```python
from build123d import *

# Parameters (mm, degrees)
SKETCH1_R           = 30
SKETCH1_R_2         = 25
BOSS_EXTRUDE1_DEPTH = 109.9
SKETCH2_W           = 5
SKETCH2_H           = 6
CUT_EXTRUDE1_DEPTH  = 31
CHAMFER1_SIZE       = 0.5


with BuildPart() as part:
    # Sketch1 → Boss-Extrude1 (new body)
    with BuildSketch(Plane.XY):
        Circle(SKETCH1_R)
        Circle(SKETCH1_R_2, mode=Mode.SUBTRACT)
    extrude(amount=BOSS_EXTRUDE1_DEPTH)

    # Sketch2 → Cut-Extrude1 (cut, through all)
    with BuildSketch(Plane(origin=(0, 0, 0), x_dir=(0, 0, -1), z_dir=(1, 0, 0))):
        with Locations((-107.4, 0)):
            Rectangle(SKETCH2_W, SKETCH2_H)
    extrude(amount=CUT_EXTRUDE1_DEPTH, mode=Mode.SUBTRACT)

    # Chamfer1
    chamfer1_edges = [part.edges().sort_by_distance(p)[0] for p in [
        (-30, 0, 109.9),
        (-30, 0, 0),
    ]]
    chamfer(chamfer1_edges, length=CHAMFER1_SIZE)


solid = part.part
```
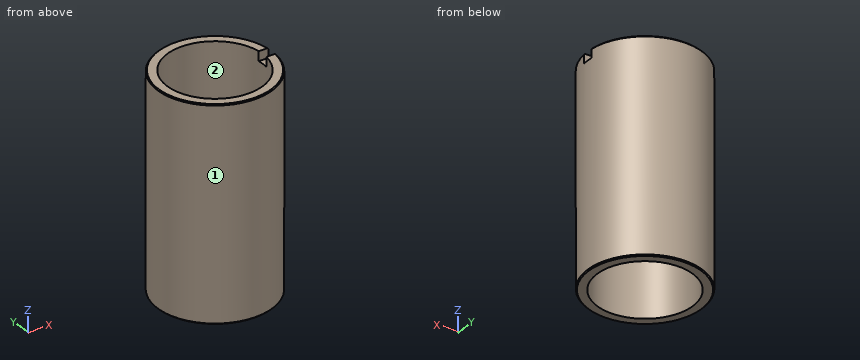
Source: CAD feature listing. Evaluate the final solid. Frame: model axes, mm. Face numbers are marked on the shaded views. Give positions to 0.01 mm unless a question says otherwise; leave off trailing zeros. Loops run counter-clockwise (first coordinate to the right, second up) from the corner with the lowest first, then second, coordinate; pieces in that order, holes last. Notation, with made-up numbers: (38.25, 24.25) -> (76.25, 24.25) arc R7 ccw to (76.25, 29.25) -> close; hole circle Ø8 at (81, 28.25). An arc over 180 degrees is marked (long way). Put each result on its own line as item: value. Start each with the question number.
1) Material intervals for probe 1 along Y at (x, z) = (0, 36); probe 2 along Y at (x, z) = (-23, 97), sorted ascending.
2) Cut plane A-A (x = 0). Return loops of the section in (y, z), then the cut area to 3 significant figures.
3) Draft query along Y for the marked faces 1 and 2. Return one class per face: released by +Y, released by -Y, zero draft, split by the parting line, or undercut.
4) Cut plane C-C (z = 61). Return loops of the section in (x, y), then the cut area to 3 significant figures.
5) Contact query for flat-ended pins moving along their axis: P1, Ø3, axis at y = 4, z = 71, coming from the -X side; P2, Ø1, axis at y = -18, z = 62, coming from the -X side; P3, Ø2.5, axis at x = 28, z = 107, coming from the +Y side. Output: stop coordinate, or through.
6) Cut plane B-B (y = 0). Return loops of the section in (x, z), then the cut area to 3 significant figures.
Results are:
1. probe 1: y = -30 to -25, 25 to 30
1. probe 2: y = -19.26 to -9.8, 9.8 to 19.26
2. outline: (-30, 0.5) -> (-29.5, 0) -> (-25, 0) -> (-25, 109.9) -> (-29.5, 109.9) -> (-30, 109.4) -> close; (25, 0) -> (29.5, 0) -> (30, 0.5) -> (30, 109.4) -> (29.5, 109.9) -> (25, 109.9) -> close
2. area: 1,100 mm2
3. face 1: split by the parting line
3. face 2: undercut
4. outline: circle Ø60 at (0, 0); hole circle Ø50 at (0, 0)
4. area: 864 mm2
5. P1: stops at x = -29.9
5. P2: stops at x = -24.37
5. P3: stops at y = 13.58
6. outline: (-30, 0.5) -> (-29.5, 0) -> (-25, 0) -> (-25, 109.9) -> (-29.5, 109.9) -> (-30, 109.4) -> close; (25, 0) -> (29.5, 0) -> (30, 0.5) -> (30, 104.9) -> (25, 104.9) -> close
6. area: 1,070 mm2
